Autodesk Inventor part; units mm, degrees
ref_plane "YZ Plane" through (0, 0, 0) normal (1, 0, 0) x (0, 1, 0)
ref_plane "XZ Plane" through (0, 0, 0) normal (0, 1, 0) x (-1, 0, 0)
ref_plane "XY Plane" through (0, 0, 0) normal (0, 0, 1) x (1, 0, 0)
sketch "Sketch1" plane through (0, 0, 0) normal (0, 0, 1) x (1, 0, 0)
  line L0 (5.08, 0) -> (45.085, 0)
  line L1 (50.165, 5.08) -> (50.165, 35.306)
  line L2 (45.085, 40.386) -> (5.08, 40.386)
  line L3 (0, 35.306) -> (0, 5.08)
  arc A0 (5.08, 40.386) -> (0, 35.306) centre (5.08, 35.306) ccw
  arc A1 (0, 5.08) -> (5.08, 0) centre (5.08, 5.08) ccw
  arc A2 (45.085, 0) -> (50.165, 5.08) centre (45.085, 5.08) ccw
  arc A3 (50.165, 35.306) -> (45.085, 40.386) centre (45.085, 35.306) ccw
  point P0 (0, 0)
  point P1 (50.165, 0)
  point P2 (50.165, 40.386)
  dimension "d0" = 50.165
  dimension "d1" = 40.386
  dimension "d2" = 5.08
extrude "Extrusion1" add sketch "Sketch1" along normal blind 7.62
sketch "Sketch2" plane through (0, 0, 7.62) normal (0, 0, 1) x (1, 0, 0)
  line L0 (0, 35.306) -> (0, 5.08)
  arc A0 (0, 5.08) -> (5.08, 0) centre (5.08, 5.08) ccw
  line L1 (5.08, 0) -> (45.085, 0)
  arc A1 (45.085, 0) -> (50.165, 5.08) centre (45.085, 5.08) ccw
  line L2 (50.165, 5.08) -> (50.165, 35.306)
  arc A2 (50.165, 35.306) -> (45.085, 40.386) centre (45.085, 35.306) ccw
  line L3 (45.085, 40.386) -> (5.08, 40.386)
  arc A3 (5.08, 40.386) -> (0, 35.306) centre (5.08, 35.306) ccw
  line L4 (45.085, 40.386) -> (5.08, 40.386)
  circle A4 centre (12.446, 31.75) radius 7.366
  line L5 (30.353, 39.116) -> (45.085, 39.116)
  line L6 (45.085, 39.116) -> (45.085, 24.384)
  line L7 (45.085, 24.384) -> (30.353, 24.384)
  line L8 (30.353, 24.384) -> (30.353, 39.116)
  line L9 (31.0509, 17.4752) -> (31.0509, 1.27)
  line L10 (31.0509, 1.27) -> (45.085, 9.3726)
  line L11 (45.085, 9.3726) -> (31.0509, 17.4752)
  circle A5 centre (12.446, 11.3013) radius 7.6835 construction
  line L12 (19.6887, 8.7364) -> (12.2447, 3.6204) construction
  line L13 (12.2447, 3.6204) -> (5.0789, 9.1192) construction
  line L14 (5.0789, 9.1192) -> (8.0941, 17.6336) construction
  line L15 (8.0941, 17.6336) -> (17.1235, 17.397) construction
  line L16 (17.1235, 17.397) -> (19.6887, 8.7364) construction
  line L17 (8.0941, 17.6336) -> (12.3737, 15.5731)
  line L18 (12.3737, 15.5731) -> (17.1235, 17.397)
  line L19 (17.1235, 17.397) -> (16.9991, 12.6499)
  line L20 (16.9991, 12.6499) -> (19.6887, 8.7364)
  line L21 (19.6887, 8.7364) -> (15.1335, 7.3908)
  line L22 (15.1335, 7.3908) -> (12.2447, 3.6204)
  line L23 (12.2447, 3.6204) -> (9.8287, 7.7099)
  line L24 (9.8287, 7.7099) -> (5.0789, 9.1192)
  line L25 (5.0789, 9.1192) -> (7.9752, 12.8838)
  line L26 (7.9752, 12.8838) -> (8.0941, 17.6336)
  point P0 (0, 0)
  dimension "d21" = 15.367
  dimension "d10" = 14.732
  dimension "d11" = 1.27
  dimension "d12" = 5.08
  dimension "d13" = 14.732
  dimension "d14" = 14.732
  dimension "d15" = 14.732
  dimension "d16" = 5.08
  dimension "d17" = 1.27
  dimension "d18" = 16.2052
  dimension "d19" = 5.08
  dimension "d20" = 1.27
  dimension "d23" = 4.7498
  dimension "d25" = 4.7498
  dimension "d26" = 4.7498
  dimension "d27" = 4.7498
  dimension "d28" = 4.7498
  dimension "d29" = 4.7498
  dimension "d30" = 4.7498
  dimension "d31" = 4.7498
  dimension "d32" = 4.747
  dimension "d33" = 3.9135
extrude "Extrusion2" cut sketch "Sketch2" against normal blind 7.62 contours A4 | L5 L6 L7 L8 | L11 L10 L9 | L17 L18 L19 L20 L21 L22 L23 L24 L25 L26
shell "Shell1" thickness 0.254 removed faces 1 at (40.407, 17.0773, 0)
properties part number "Passenger Base EM" material "Wood (Birch)"
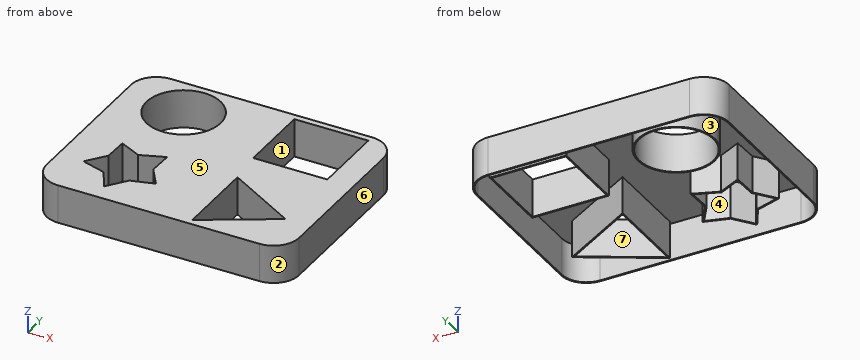
Geometry: final body of the model. Coordinates: model frame, mm. Face numbers are marked on the shaded views. A direction names the side the tool comes from. Give positions to 0.01 mm unless a question says otherwise; leave off trailing zeros. Write each loop counter-clockwise with the first axis right and the second up, starting at its lowest first coordinate (ties: lowest second). Pieces come first, ordered by that corner, then holes. Notation, with made-up numbers: M 44.5,-19 L 49.5,-19 A27 cw 49.5,11 Z; hole C 0,71.5 d5. An arc over 180 degrees is marked long. Answer in a Markdown table with one row per item. Add a question column.
(1) Section B-B on x = 34. Return loops of the section in (y, z).
(2) Reachability of the marked faces 1, 2 and 3 from +Z, -Z, +X, -X, +Y, -Y: full face, straight path, thin tool, end or side. Return the list, or none.
(3) Section D-D on x = 22.5. Return loops of the section in (y, z).
(4) Section A-A on y = 31.75. Return loops of the section in (x, z) (3 decimals).
(5) Mould query, pull axis X, two halves, no side actions, for the marked faces 4, 5, 6 and 7. Classes: +X half, -X half, draft (parallel to the pull), parting line (faces both ways), or undercut.
(6) First-contact query: pin 1 (2 mm diameter, centred on x = 8.5, z = 5.5, fed in from -Y). Flat tip, straight axial feed; report the tip coordinate or a pass-through.
(7) Ray query, line 1 (X direction, y = 27, z = 5.5) (3 decimals); line 2 (Y direction, x = 44, z = 5.25); line 3 (X direction, y = 12, z = 3) (3 decimals). Return the intervals inside material, ascending.
(8) Section C-C on z = 6.75. State how many separate pieces and enclosed holes the cut face has, and give its area (3 significant figures).
Result set:
| question | item | result |
|---|---|---|
| 1 | outline | M 0,0 L 0.25,0 L 0.25,7.37 L 2.68,7.37 L 2.68,0 L 2.97,0 L 2.97,7.62 L 0,7.62 Z; M 15.77,0 L 16.07,0 L 16.07,7.37 L 24.13,7.37 L 24.13,0 L 24.38,0 L 24.38,7.62 L 15.77,7.62 Z; M 39.12,0 L 39.37,0 L 39.37,7.37 L 40.13,7.37 L 40.13,0 L 40.39,0 L 40.39,7.62 L 39.12,7.62 Z |
| 2 | face 1 | +Z, -Z |
| 2 | face 2 | +Z, -Z, +X, -Y |
| 2 | face 3 | -Z |
| 3 | outline | M 0,0 L 0.25,0 L 0.25,7.37 L 40.13,7.37 L 40.13,0 L 40.39,0 L 40.39,7.62 L 0,7.62 Z |
| 4 | outline | M 0,0 L 0.254,0 L 0.254,7.366 L 4.826,7.366 L 4.826,0 L 5.08,0 L 5.08,7.62 L 0,7.62 Z; M 19.812,0 L 20.066,0 L 20.066,7.366 L 30.099,7.366 L 30.099,0 L 30.353,0 L 30.353,7.62 L 19.812,7.62 Z; M 45.085,0 L 45.339,0 L 45.339,7.366 L 49.911,7.366 L 49.911,0 L 50.165,0 L 50.165,7.62 L 45.085,7.62 Z |
| 5 | face 4 | undercut |
| 5 | face 5 | draft |
| 5 | face 6 | +X half |
| 5 | face 7 | undercut |
| 6 | pin 1 | stops at y = 0 |
| 7 | line 1 | x = 0 to 0.254, 6.488 to 6.816, 18.076 to 18.404, 30.099 to 30.353, 45.085 to 45.339, 49.911 to 50.165 |
| 7 | line 2 | y = 0 to 0.25, 8.45 to 8.75, 10 to 10.29, 24.13 to 24.38, 39.12 to 39.37, 40.13 to 40.39 |
| 7 | line 3 | x = 0 to 0.254, 6.975 to 7.295, 17.446 to 17.754, 30.797 to 31.051, 40.534 to 41.042, 49.911 to 50.165 |
| 8 | separate pieces | 5 |
| 8 | enclosed holes | 5 |
| 8 | area | 96.0 mm^2 |
